Could you check a few things on this model? Use its own coordinates, in mm. A direction names the side the tool comes from. Coordinates: 2 decimals unless noted, no trailing zeros. Write each loop counter-clockwise with the first axis right and the second up, starting at its lowest first coordinate (ties: lowest second). Pieces come first, ordered by that corner, then holes. Notation, with made-up numbers: M 8,88 L 50,88 A23 ccw 50,113 Z; hole C -6,-30 d11. An arc over 180 degrees is marked long. Answer as CSV lines item,"result". Start each with the question number.
Item 1: On a 3-axis mill with a long thin cutter (end or side, diameter ignored), from which of +Z, -Z, +X, -X, +Y, -Y can I reach the whole of each face in a straight line? I mean faces 5 (the flat face through (16, -4.826, 20)), 6 (the cylindrical face through (73.02, -0.42, 7.78)). Say none if no direction works.
Item 2: Suppose I cut it at C-C, the plane z = 4. State how many separate pieces and enclosed holes the cut face has, and give its area (3 significant figures).
Item 3: We'd pull the mould along X, two halves only. Please class faces 1 (the flat face through (11, -11, 40.234)), 2 (the flat face through (18.529, 0, 20)), 3 (the cylindrical face through (4.8, 26.77, 39.24)), 4 (the cylindrical face through (43.825, 0.447, 7.776)): +X half, -X half, draft (parallel to the pull), parting line (faces both ways), or undercut.
Item 4: I'm going to push flat-ended pins straight in: P1, Ø10, axis at y = -1.5, z = 17, coming from the -X side (3 decimals); P2, Ø10, axis at y = -7, z = 14.5, coming from the -X side; P3, Ø12, axis at x = 11, z = 18.5, coming from the +Y side. Where does each tip first touch, or does it pass through?
Item 5: Suppose I cut it at B-B, the plane x = 62.5. Write out the boundary of the cut face in (y, z), and give its area (3 significant figures).
Item 6: If I drill on line 1 along Y through (x, z) = (-7, 25); line 2 along Z through (x, y) = (37, -20); line 3 along Y through (x, z) = (-4.5, 11), over which ranges is the centre line in solid material (lowest first)? Write a range as [from, to].
```python
from build123d import *

# Parameters (mm, degrees)
F0_R        = 10.16
F1_DEPTH    = 15.7734
F2_DEPTH    = 40.2336
F3_T1_DEPTH = 37.9988318329
F3_T3_DEPTH = 37.9988318329
F3_T6_ANGLE = 213.1574660215
F3_T8_ANGLE = 173.1044855741


# Not quite as in the source:
# - a fillet or chamfer that OpenCascade refuses, or shapes differently, is made with other operations: its cross-section is extruded or revolved along the edge and cut away or added


with BuildPart() as f1:
    # F0 (on Top) → F1 (new body)
    with BuildSketch(Plane.XY):
        with BuildLine():
            Line((53.975, 19.05), (9.780704698, 26.8489932886))
            ThreePointArc((9.780704698, 26.8489932886), (23.4095521288, 16.3866864902), (28.575, 0))
            ThreePointArc((28.575, 0), (23.4095521288, -16.3866864902), (9.780704698, -26.8489932886))
            Line((9.780704698, -26.8489932886), (53.975, -19.05))
            ThreePointArc((53.975, -19.05), (73.025, 0), (53.975, 19.05))
        make_face()
        with Locations((53.975, 0)):
            Circle(F0_R, mode=Mode.SUBTRACT)
    extrude(amount=F1_DEPTH)

    # F0 (on Top) → F2 (join)
    with BuildSketch(Plane.XY):
        with BuildLine():
            Line((9.780704698, 26.8489932886), (0, 28.575))
            ThreePointArc((0, 28.575), (-28.575, 0), (0, -28.575))
            Line((0, -28.575), (9.780704698, -26.8489932886))
            ThreePointArc((9.780704698, -26.8489932886), (23.4095521288, -16.3866864902), (28.575, 0))
            ThreePointArc((28.575, 0), (23.4095521288, 16.3866864902), (9.780704698, 26.8489932886))
        make_face()
        with BuildLine():
            ThreePointArc((-13.4477648793, 4.826), (-8.2213496839, 11.6851215494), (0, 14.2875))
            ThreePointArc((0, 14.2875), (8.2213496839, 11.6851215494), (13.4477648793, 4.826))
            Line((13.4477648793, 4.826), (18.5293, 4.826))
            Line((18.5293, 4.826), (18.5293, -4.826))
            Line((18.5293, -4.826), (13.4477648793, -4.826))
            ThreePointArc((13.4477648793, -4.826), (0, -14.2875), (-13.4477648793, -4.826))
            Line((-13.4477648793, -4.826), (-18.5293, -4.826))
            Line((-18.5293, -4.826), (-18.5293, 4.826))
            Line((-18.5293, 4.826), (-13.4477648793, 4.826))
        make_face(mode=Mode.SUBTRACT)
        with BuildLine():
            ThreePointArc((-13.4477648793, -4.826), (-14.2875, 0), (-13.4477648793, 4.826))
            Line((-13.4477648793, 4.826), (-18.5293, 4.826))
            Line((-18.5293, 4.826), (-18.5293, -4.826))
            Line((-18.5293, -4.826), (-13.4477648793, -4.826))
        make_face()
    extrude(amount=F2_DEPTH)

    # F3: fillet of radius 3.302 on 4 edges, made by hand

    # F3_s2 → F3_t1 (cut)
    with BuildSketch(Plane(origin=(18.7103124217, -3.3018198391, 0), x_dir=(0, 0, 1), z_dir=(-0.9847835588, 0.1737853339, 0))):
        with BuildLine():
            ThreePointArc((36.9316, 28.1401901932), (39.2664665915, 27.1730567847), (40.2336, 24.8381901932))
            Line((40.2336, 24.8381901932), (40.2336, 28.1401901932))
            Line((40.2336, 28.1401901932), (36.9316, 28.1401901932))
        make_face()
    extrude(amount=F3_T1_DEPTH, mode=Mode.SUBTRACT)

    # F3_s4 → F3_t3 (cut)
    with BuildSketch(Plane(origin=(-18.7103124217, -3.3018198391, 0), x_dir=(0, 0, 1), z_dir=(0.9847835588, 0.1737853339, 0))):
        with BuildLine():
            ThreePointArc((36.9316, 28.1401901932), (39.2664665915, 27.1730567847), (40.2336, 24.8381901932))
            Line((40.2336, 24.8381901932), (40.2336, 28.1401901932))
            Line((40.2336, 28.1401901932), (36.9316, 28.1401901932))
        make_face()
    extrude(amount=F3_T3_DEPTH, mode=Mode.SUBTRACT)

    # F3_s5 → F3_t6 (revolve, cut)
    with BuildSketch(Plane(origin=(0, 0, 0), x_dir=(0, 0, 1), z_dir=(0.95842855, -0.2853326385, 0))):
        with BuildLine():
            ThreePointArc((40.2336, -25.273), (39.2664665915, -27.6078665915), (36.9316, -28.575))
            Line((36.9316, -28.575), (40.2336, -28.575))
            Line((40.2336, -28.575), (40.2336, -25.273))
        make_face()
    revolve(axis=Axis((0, 0, 40.2336), (0, 0, 1)), revolution_arc=F3_T6_ANGLE, mode=Mode.SUBTRACT)

    # F3_s7 → F3_t8 (revolve, cut)
    with BuildSketch(Plane(origin=(0, 0, 0), x_dir=(0, 0, 1), z_dir=(-0.9981900481, -0.0601384063, 0))):
        with BuildLine():
            ThreePointArc((36.9316, -28.575), (39.2664665915, -27.6078665915), (40.2336, -25.273))
            Line((40.2336, -25.273), (40.2336, -28.575))
            Line((40.2336, -28.575), (36.9316, -28.575))
        make_face()
    revolve(axis=Axis((0, 0, 40.2336), (0, 0, 1)), revolution_arc=F3_T8_ANGLE, mode=Mode.SUBTRACT)


solid = f1.part
```
Ans:
1,face 5,"+Z, -Z"
1,face 6,"+Z, -Z, +X"
2,separate pieces,"1"
2,enclosed holes,"2"
2,area,"3,410 mm^2"
3,face 1,"draft"
3,face 2,"undercut"
3,face 3,"+X half"
3,face 4,"undercut"
4,P1,"stops at x = -28.575"
4,P2,"stops at x = -28.5"
4,P3,"stops at y = 27.69"
5,outline,"M -17.04,0 L -5.53,0 L -5.53,15.77 L -17.04,15.77 Z; M 5.53,0 L 17.04,0 L 17.04,15.77 L 5.53,15.77 Z"
5,area,"363 mm^2"
6,line 1,"y = [-27.7, -12.46], [12.46, 27.7]"
6,line 2,"z = [0, 15.77]"
6,line 3,"y = [-28.22, -13.56], [13.56, 28.22]"
